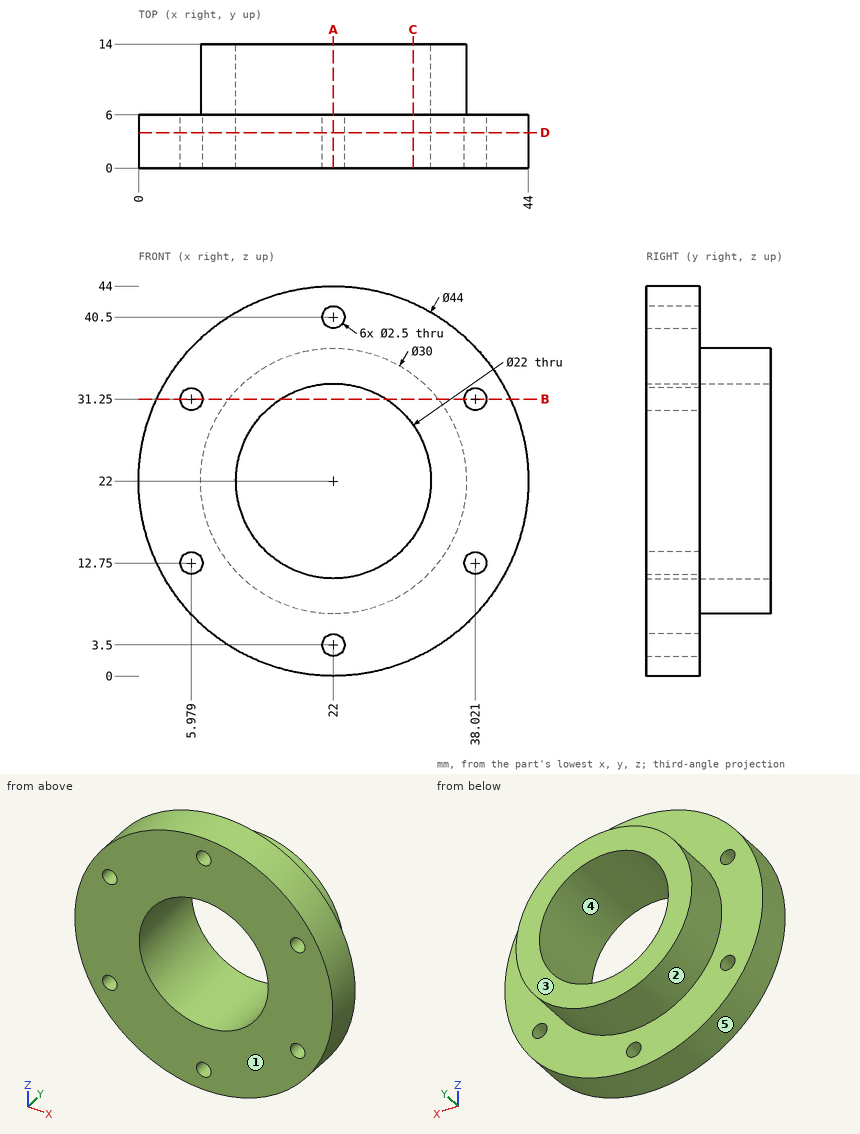
Geometry check sheet. Reference: drawing and pictorial views, mm from the part's lowest x, y, z. A direction names the side the tool comes from. Coordinates: 2 decimals unless noted, no trailing zeros. Loops run counter-clockwise (first coordinate to the right, second up) from the corner with the lowest first, then second, coordinate; pieces in that order, holes last.
1) Sectioned sample at A-A (x = 22). Record the boundary of the cut face in (y, z).
2) Access from +Z, -Z, +X, -X, +Y, -Y to the whole of each face (thin tool, end or side, straight path). Record for the marked faces 1 and 2.
3) Sectioned sample at D-D (y = 4). Record the boundary of the cut face in (x, z).
4) Sectioned sample at C-C (x = 31). Record the boundary of the cut face in (y, z) (1 decimal).
5) Material ranges on probe 1 along X at (y, z) = (8, 21.5); probe 2 along X at (y, z) = (3, 22); probe 3 along Y at (x, z) = (19, 39), recorded low to high.
6) Sectioned sample at B-B (z = 31.25). Record the boundary of the cut face in (x, y), and give its area (3 significant figures).
7) Release check for a two-part mould opening along Z. For the marked faces 3, 4 and 5 record: released by +Z, released by -Z, zero draft, split by the parting line, or undercut.
8) Gauge pin test, flat ends, axial feed: pin 1 (1.5 mm diameter, centred on y = 10, z = 22, fed in from -X); pin 2 (3 mm diameter, centred on x = 22, z = 40.5, fed in from +Y); pin 3 (3 mm diameter, centred on y = 9, z = 17.5, fed in from +X). Record the tip position at first contact, or that the pin passes through.
Check sheet entries:
1. outline: (0, 0) - (6, 0) - (6, 2.25) - (0, 2.25) - close; (0, 4.75) - (6, 4.75) - (6, 7) - (14, 7) - (14, 11) - (0, 11) - close; (0, 33) - (14, 33) - (14, 37) - (6, 37) - (6, 39.25) - (0, 39.25) - close; (0, 41.75) - (6, 41.75) - (6, 44) - (0, 44) - close
2. face 1: +Z, -Z, +X, -X, -Y
2. face 2: +Y
3. outline: circle Ø44 at (22, 22); hole circle Ø2.5 at (5.98, 12.75); hole circle Ø2.5 at (5.98, 31.25); hole circle Ø22 at (22, 22); hole circle Ø2.5 at (22, 3.5); hole circle Ø2.5 at (22, 40.5); hole circle Ø2.5 at (38.02, 12.75); hole circle Ø2.5 at (38.02, 31.25)
4. outline: (0, 1.9) - (6, 1.9) - (6, 10) - (14, 10) - (14, 15.7) - (0, 15.7) - close; (0, 28.3) - (14, 28.3) - (14, 34) - (6, 34) - (6, 42.1) - (0, 42.1) - close
5. probe 1: x = 7.01 to 11.01, 32.99 to 36.99
5. probe 2: x = 0 to 11, 33 to 44
5. probe 3: y = 0 to 6
6. outline: (2.04, 0) - (4.73, 0) - (4.73, 6) - (2.04, 6) - close; (7.23, 0) - (16.05, 0) - (16.05, 14) - (10.19, 14) - (10.19, 6) - (7.23, 6) - close; (27.95, 0) - (36.77, 0) - (36.77, 6) - (33.81, 6) - (33.81, 14) - (27.95, 14) - close; (39.27, 0) - (41.96, 0) - (41.96, 6) - (39.27, 6) - close
6. area: 232 mm2
7. face 3: zero draft
7. face 4: undercut
7. face 5: split by the parting line
8. pin 1: stops at x = 7
8. pin 2: stops at y = 6
8. pin 3: stops at x = 36.7
